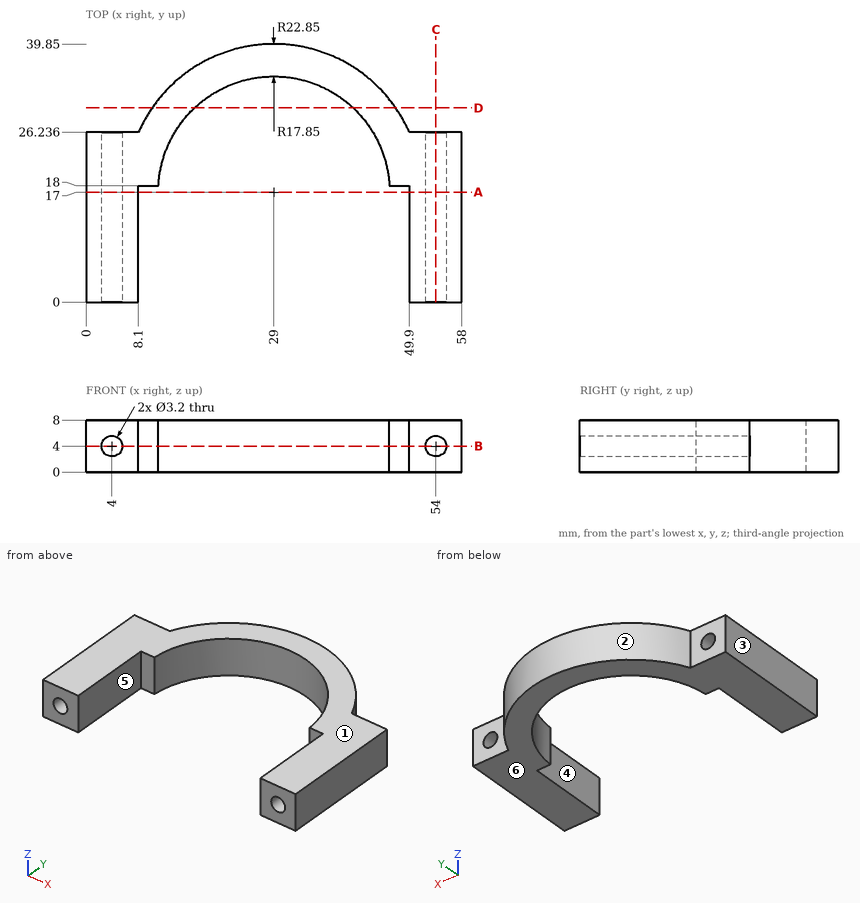
Job drawing, mm, ordinate dimensions from the low corner. One solid piece. A direction names the side the tool comes from. Give positions to 0.01 mm unless a question says otherwise; leave off trailing zeros. Loops run counter-clockwise (first coordinate to the right, second up) from the corner with the lowest first, then second, coordinate; pieces in that order, holes last. Notation, with made-up numbers: M 83.25,54 L 122.25,54 A26 cw 122.25,87 Z; hole C 22.25,-35.5 d7. An arc over 180 degrees is marked long. Answer in a Markdown table with one row per item. Add a question column.
Item 1: Tool access for the marked faces 5 and 6: list every direction of +Z, -Z, +X, -X, +Y, -Y with a clear straight run to the whole face (end or side of a thin tool).
Item 2: Mould opens along X. For the marked faces 1, 2, 3 and 4 say: +X half, -X half, draft (parallel to the pull), parting line (faces both ways), or undercut.
Item 3: Band-saw the part on D-D on y = 30. Give the cut face in (x, z), then the cut area to 3 significant figures.
Item 4: Band-saw the part on A-A on y = 17. Give the cut face in (x, z).
Item 5: Probe probe 1 along X at (y, z) = (11.75, 4); probe 2 along Z at (x, y) = (54, 18.25); probe 3 along X at (y, z) = (20.5, 4). List the from-to ranges inside material, lowest first.
Item 6: Band-saw the part on B-B on z = 4. Give the cut face in (x, y).
Item 7: Band-saw the part on C-C on x = 54. Give the cut face in (y, z).
Item 8: Drop flat-ended pins along their axis: P1, Ø4, axis at x = 22, z = 4.5, coming from the +Y side; P2, Ø1.5, axis at x = 48.5, y = 29.5, coming from the -Z side; P3, Ø1.5, axis at x = 9, z = 3, coming from the -Y side; P4, Ø3, axis at y = 35.5, z = 5, coming from the +X side. Give the stop position or say it passes through.
Reply:
| question | item | result |
|---|---|---|
| 1 | face 5 | +Z, -Z, -Y |
| 1 | face 6 | -Z, +X, -X, +Y, -Y |
| 2 | face 1 | draft |
| 2 | face 2 | parting line |
| 2 | face 3 | -X half |
| 2 | face 4 | undercut |
| 3 | outline | M 10.21,0 L 16.77,0 L 16.77,8 L 10.21,8 Z; M 41.23,0 L 47.79,0 L 47.79,8 L 41.23,8 Z |
| 3 | area | 105 mm^2 |
| 4 | outline | M 0,0 L 8.1,0 L 8.1,8 L 0,8 Z; M 49.9,0 L 58,0 L 58,8 L 49.9,8 Z; hole C 4,4 d3.2; hole C 54,4 d3.2 |
| 5 | probe 1 | x = 0 to 2.4, 5.6 to 8.1, 49.9 to 52.4, 55.6 to 58 |
| 5 | probe 2 | z = 0 to 2.4, 5.6 to 8 |
| 5 | probe 3 | x = 0 to 2.4, 5.6 to 11.5, 46.5 to 52.4, 55.6 to 58 |
| 6 | outline | M 0,0 L 2.4,0 L 2.4,26.24 L 0,26.24 Z; M 5.6,0 L 8.1,0 L 8.1,18 L 11.18,18 A17.85 cw 46.82,18 L 49.9,18 L 49.9,0 L 52.4,0 L 52.4,26.24 L 49.9,26.24 A22.85 ccw 8.1,26.24 L 5.6,26.24 Z; M 55.6,0 L 58,0 L 58,26.24 L 55.6,26.24 Z |
| 7 | outline | M 0,0 L 26.24,0 L 26.24,2.4 L 0,2.4 Z; M 0,5.6 L 26.24,5.6 L 26.24,8 L 0,8 Z |
| 8 | P1 | stops at y = 39.3 |
| 8 | P2 | stops at z = 0 |
| 8 | P3 | stops at y = 18 |
| 8 | P4 | stops at x = 44.27 |
